```python
from build123d import *

# Parameters (mm, degrees)
ESQUISSE1_R                  = 12.5
BASE_EXTRUSION_DEPTH         = 121
ESQUISSE2_R                  = 10
ENL_V_MAT_EXTRU_1_DEPTH      = 58
ESQUISSE3_R                  = 4
ENL_V_MAT_EXTRU_2_DEPTH      = 66.433172015
ENL_V_MAT_EXTRU_3_DEPTH      = 15
ENL_V_MAT_EXTRU_3_DEPTH_BACK = 8
ESQUISSE4_R                  = 5
ESQUISSE5_R                  = 3
ENL_V_MAT_EXTRU_4_DEPTH      = 124.35923164
ESQUISSE9_W                  = 55
ESQUISSE9_H                  = 32.337681811
ENL_V_MAT_EXTRU_6_DEPTH      = 123.284504453
ESQUISSE6_W                  = 1.5
ESQUISSE6_H                  = 2


with BuildPart() as part:
    # Esquisse1 → Base-Extrusion (new body)
    with BuildSketch(Plane.XY):
        with Locations(Location((0, 0, 0), (0, 0, 180))):
            Circle(ESQUISSE1_R)
    extrude(amount=BASE_EXTRUSION_DEPTH)

    # Esquisse2 → Enlèv. mat.-Extru.1 (cut)
    with BuildSketch(Plane.XY.offset(121)):
        Circle(ESQUISSE2_R)
    extrude(amount=-ENL_V_MAT_EXTRU_1_DEPTH, mode=Mode.SUBTRACT)

    # Esquisse3 → Enlèv. mat.-Extru.2 (cut, through all)
    with BuildSketch(Plane.XY.offset(63)):
        Circle(ESQUISSE3_R)
    extrude(amount=-ENL_V_MAT_EXTRU_2_DEPTH, mode=Mode.SUBTRACT)

    # Esquisse4 → Enlèv. mat.-Extru.3 (cut, two sides: drawn at the far end of the back side and taken through both)
    with BuildSketch(Plane(origin=(0, 0, 0), x_dir=(-1, 0, 0), z_dir=(0, 1, 0)).offset(-ENL_V_MAT_EXTRU_3_DEPTH_BACK)):
        with Locations(Location((0, 56, 0), (0, 0, 90))):
            Circle(ESQUISSE4_R)
    extrude(amount=ENL_V_MAT_EXTRU_3_DEPTH + ENL_V_MAT_EXTRU_3_DEPTH_BACK, mode=Mode.SUBTRACT)

    # Esquisse5 → Enlèv. mat.-Extru.4 (cut, through all)
    with BuildSketch(Plane(origin=(0, -8, 0), x_dir=(-1, 0, 0), z_dir=(0, 1, 0))):
        with Locations(Location((0, 56, 0), (0, 0, 90))):
            Circle(ESQUISSE5_R)
    extrude(amount=-ENL_V_MAT_EXTRU_4_DEPTH, mode=Mode.SUBTRACT)

    # Esquisse9 → Enlèv. mat.-Extru.6 (cut, through all)
    with BuildSketch(Plane(origin=(0, 0, 0), x_dir=(0, 0, -1), z_dir=(1, 0, 0))):
        with Locations((-98.5, 16.168840906)):
            Rectangle(ESQUISSE9_W, ESQUISSE9_H)
    extrude(amount=-ENL_V_MAT_EXTRU_6_DEPTH, mode=Mode.SUBTRACT)

    # Esquisse6 → Anneau élastique (revolve)
    with BuildSketch(Plane(origin=(0, 0, 0), x_dir=(0, 0, -1), z_dir=(1, 0, 0)), mode=Mode.PRIVATE) as anneau_lastique_sk:
        with Locations((-119.25, 9)):
            Rectangle(ESQUISSE6_W, ESQUISSE6_H)
    revolve(anneau_lastique_sk.sketch.rotate(Axis((0, 0, -6.276986183), (0, 0, 1)), 270), axis=Axis((0, 0, -6.276986183), (0, 0, 1)))


solid = part.part
```
Part model, mm, in its own coordinate system. A direction names the side the tool comes from. Round coordinates to 2 decimals unless told otherwise and drop trailing zeros. Order: outer loops, then holes, each group sorted by start corner. A loop starts at its lowest first (then second) coordinate and runs counter-clockwise, first axis right, second up. Notation, with made-up numbers: M 25,37 L 62,37 A25 cw 62,66 Z; hole C 69.25,34 d3. An arc over 180 degrees is marked long. Put each result on its own line as item: value. Start each with the question number.
1. Slice it at C-C on z = 11. List the corners of the cut face in (x, y), then the cut area to 3 significant figures.
2. Tool access for faces 5 (the face through (0, 11, 96)), 6 (the face through (0, 8.2, 118.5)), 7 (the face through (-0.521, 3.966, 61.472)), 8 (the face through (0, 8.2, 120)), 9 (the face through (4, 2, 59)): list every direction of +Z, -Z, +X, -X, +Y, -Y with a clear straight run to the whole face (end or side of a thin tool).
3. Slice it at D-D on z = 99. List the corners of the cut face in (x, y).
4. Slice it at A-A on y = 6. List the corners of the cut face in (x, z).
5. Drop flat-ended pins along their axis: pin 1 (3 mm diameter, centred on x = -6, z = 87.5, fed in from +Y); pin 2 (3 mm diameter, centred on y = 10.5, z = 94, fed in from -X); pin 3 (1.2 mm diameter, centred on x = -11.5, z = 99, fed in from +Y). Give the stop position or say it passes through.
6. Slice it at B-B on z = 56. List the corners of the cut face in (x, y).
7. Two-plate mould, pull along Z, no slides. Class faces 1 (the face through (3, -3, 0)), 2 (the face through (0.1, -8, 59.3)), 3 (the face through (-0.1, -4.3, 63)), 4 (the face through (-6.99, 7.15, 119.24)): +Z half, -Z half, draft (parallel to the pull), parting line (faces both ways), or undercut.
8. Drill centre lines: probe 1 along Z at (x, y) = (-3.5, 9); probe 2 along X at (y, z) = (-3, 19); probe 3 along X at (y, z) = (7.5, 40.5). Where is each one in solid material? Low to high. Write a range as [from, to].
Findings:
1. outline: C 0,0 d25; hole C 0,0 d8
1. area: 441 mm2
2. face 5: +Z, -X, +Y
2. face 6: none
2. face 7: +Z, -Z
2. face 8: +Z
2. face 9: +Y
3. outline: M -12.5,0 A12.5 ccw long 0,12.5 L 0,10 A10 cw long -10,0 Z
4. outline: M -10.97,0 L 10.97,0 L 10.97,121 L 8,121 L 8,120 L 5.29,120 L 5.29,118.5 L 8,118.5 L 8,63 L -8,63 L -8,71 L -10.97,71 Z; M -8,118.5 L -5.29,118.5 L -5.29,120 L -8,120 Z; hole C 0,56 d10
5. pin 1: y = -6.61
5. pin 2: x = 0
5. pin 3: y = 0
6. outline: M -5,-8 L -5,11.46 A12.5 ccw -3,-12.13 L -3,-8 Z; M 3,-12.13 A12.5 ccw 5,11.46 L 5,-8 L 3,-8 Z
7. face 1: -Z half
7. face 2: undercut
7. face 3: undercut
7. face 4: draft
8. probe 1: [0, 52.43], [59.57, 63], [118.5, 120]
8. probe 2: [-12.13, -2.65], [2.65, 12.13]
8. probe 3: [-10, 10]
